from build123d import *

# Parameters (mm, degrees)
F0_R     = 0.3
F0_W     = 5
F0_H     = 0.3
F1_DEPTH = 17
F2_DEPTH = 0.75
F3_DEPTH = 6.1


# Not quite as in the source:
# - a feature names something its author has since deleted; it is built from what else it names


with BuildPart() as f1:
    # F0 (on Top) → F1 (new body)
    with BuildSketch(Plane.XY):
        Polygon((12.1, -11.1), (16.85, -11.1), (16.85, 11.1), (12.1, 11.1), (12.1, 10.8), (7.1, 10.8), (7.1, 11.1), (-7.1, 11.1), (-7.1, 10.8), (-12.1, 10.8), (-12.1, 11.1), (-16.85, 11.1), (-16.85, -11.1), (-12.1, -11.1), (-12.1, -10.8), (-7.1, -10.8), (-7.1, -11.1), (7.1, -11.1), (7.1, -10.8), (12.1, -10.8), align=None)
        with Locations((-14, -7.62)):
            Circle(F0_R, mode=Mode.SUBTRACT)
        with Locations((-14, 7.62)):
            Circle(F0_R, mode=Mode.SUBTRACT)
        with Locations((14, 0)):
            Circle(F0_R, mode=Mode.SUBTRACT)
        with Locations((14, 7.62)):
            Circle(F0_R, mode=Mode.SUBTRACT)
        with Locations((-9.6, 10.95)):
            Rectangle(F0_W, F0_H)
        with Locations((9.6, 10.95)):
            Rectangle(F0_W, F0_H)
        with Locations((9.6, -10.95)):
            Rectangle(F0_W, F0_H)
        with Locations((-9.6, -10.95)):
            Rectangle(F0_W, F0_H)
        with Locations((-14, -7.62)):
            Circle(F0_R)
        with Locations((-14, 7.62)):
            Circle(F0_R)
        with Locations((14, 0)):
            Circle(F0_R)
        with Locations((14, 7.62)):
            Circle(F0_R)
    extrude(amount=F1_DEPTH)

    # F0 (on Top) → F2 (join)
    with BuildSketch(Plane.XY):
        with Locations((9.6, 10.95)):
            Rectangle(F0_W, F0_H)
        with Locations((-9.6, 10.95)):
            Rectangle(F0_W, F0_H)
        with Locations((-9.6, -10.95)):
            Rectangle(F0_W, F0_H)
        with Locations((9.6, -10.95)):
            Rectangle(F0_W, F0_H)
    extrude(amount=-F2_DEPTH)

    # F0 (on Top) → F3 (join)
    with BuildSketch(Plane.XY):
        with Locations((14, 0)):
            Circle(F0_R)
        with Locations((-14, 7.62)):
            Circle(F0_R)
        with Locations((-14, -7.62)):
            Circle(F0_R)
        with Locations((14, 7.62)):
            Circle(F0_R)
    extrude(amount=-F3_DEPTH)


solid = f1.part
Input: part model. Units: mm. Frame: model coordinates. Give positions to 0.01 mm unless a question says otherwise; leave off trailing zeros. Order: outer loops, then holes, each group sorted by start corner. A loop starts at its lowest first (then second) coordinate and runs counter-clockwise, first axis right, second up. Notation, with made-up numbers: (-17, 11.25) - (14, 11.25) arc R15 ccw to (14, 38.25) - close; hole circle Ø2 at (-11, -0.5). An arc over 180 degrees is marked (long way). Answer as a JSON object with one key per item and string values. Group by question number.
Q1. Cut plane C-C, the plane y = -4.5. Output: boundary loops of the cut face in (x, z).
Q2. Cut plane A-A, the plane x = 9.5. Output: boundary loops of the cut face in (y, z), then the cut area to 3 significant figures.
Q3. Line query: probe 1 along Z at (x, y) = (-13.5, -2.25); probe 2 along X at (y, z) = (-7.5, -4). Output: solid intervals per line, ascending.
Q4. First-contact query: pin 1 Ø5 at (x, y) = (3.5, -0.5) entering from -Z. Flat tip, straight axial feed; report the tip coordinate or a pass-through.
Q5. Cut plane B-B, the plane z = -3.5. Output: boundary loops of the cut face in (x, y), then the cut area to 3 significant figures.
Q6. Mould query, pull axis Y, two halves, no side actions, for faces 1 (the face through (0, 11.1, 8)), 2 (the face through (0, -11.1, 8)), 3 (the face through (0, 0, 0)), 4 (the face through (0, 0, 17)). Classes: pulls with the +Y half, pulls with the -Y half, needs draft (parallel to the pull), parting line crosses it, or undercut.
Results:
{
 "1": {"outline": "(-16.85, 0) - (16.85, 0) - (16.85, 17) - (-16.85, 17) - close"},
 "2": {"outline": "(-11.1, -0.75) - (-10.8, -0.75) - (-10.8, 0) - (10.8, 0) - (10.8, -0.75) - (11.1, -0.75) - (11.1, 17) - (-11.1, 17) - close", "area": "378 mm^2"},
 "3": {"probe 1": "0 to 17", "probe 2": "-14.27 to -13.73"},
 "4": {"pin 1": "z = 0"},
 "5": {"outline": "circle Ø0.6 at (-14, -7.62); circle Ø0.6 at (-14, 7.62); circle Ø0.6 at (14, 0); circle Ø0.6 at (14, 7.62)", "area": "1.13 mm^2"},
 "6": {"face 1": "pulls with the +Y half", "face 2": "pulls with the -Y half", "face 3": "undercut", "face 4": "needs draft"}
}
